Build history of the part. All positions in model axes, mm. A direction names the side the tool comes from. Give positions to 0.01 mm unless a question says otherwise; leave off trailing zeros. Write each loop counter-clockwise with the first axis right and the second up, starting at its lowest first coordinate (ties: lowest second). Pieces come first, ordered by that corner, then holes. Notation, with made-up numbers: M -13,81 L 37,81 A18 ccw 37,88 Z; hole C 88,76 d8. An arc over 180 degrees is marked long. Return JSON: item names as keys, results as strings. Group by question number.
Q1. Band-saw the part on B-B, the plane x = 0. Give the cut face in (y, z).
Q2. Band-saw the part on C-C, the plane z = -0.65. Give the cut face in (x, y).
Q3. Band-saw the part on A-A, the plane y = -22.5. Give the cut face in (x, z).
Q4. Tool access for faces 1 (the flat face through (0, 0, 0)), 2 (the cylindrical face through (0.45, -2.37, 1.43)): list every direction of +Z, -Z, +X, -X, +Y, -Y with a clear straight run to the whole face (end or side of a thin tool).
Q5. Flat gauge pins, fed straight in: pin 1 Ø0.7 at (x, y) = (-1, -19) entering from +Z; pin 2 Ø0.7 at (x, y) = (-1, -21.5) entering from -Z. Where does each tip first touch, or does it go through?
Q6. Wall check: probe 1 along Z at (x, y) = (1, -11.5); probe 2 along Y at (x, z) = (0.2, -0.85); probe 3 along Y at (x, z) = (-0.3, -1.5). Give the ranges that are in metal, low to high.
from build123d import *

# Parameters (mm, degrees)
SKETCH1_R           = 1.5
BOSS_EXTRUDE1_DEPTH = 4.8
SKETCH2_R           = 1.7
BOSS_EXTRUDE2_DEPTH = 1.2
SKETCH3_W           = 0.6
SKETCH3_H           = 0.4
BOSS_EXTRUDE3_DEPTH = 27


with BuildPart() as part:
    # Sketch1 → Boss-Extrude1 (new body)
    with BuildSketch(Plane(origin=(0, 0, 0), x_dir=(1, 0, 0), z_dir=(0, 1, 0))):
        with Locations(Location((0, 0, 0), (0, 0, 270))):
            Circle(SKETCH1_R)
    extrude(amount=-BOSS_EXTRUDE1_DEPTH)

    # Sketch2 → Boss-Extrude2 (add)
    with BuildSketch(Plane.XZ.offset(4.8)):
        with Locations(Location((0, 0, 0), (0, 0, 270))):
            Circle(SKETCH2_R)
    extrude(amount=BOSS_EXTRUDE2_DEPTH)

    # Sketch3 → Boss-Extrude3 (add)
    with BuildSketch(Plane.XZ.offset(6)):
        with Locations((-1.27, 0)):
            Rectangle(SKETCH3_W, SKETCH3_H)
        with Locations((1.27, 0)):
            Rectangle(SKETCH3_W, SKETCH3_H)
    extrude(amount=BOSS_EXTRUDE3_DEPTH)


solid = part.part
From the geometry:
{
 "1": {"outline": "M -6,-1.7 L -4.8,-1.7 L -4.8,-1.5 L 0,-1.5 L 0,1.5 L -4.8,1.5 L -4.8,1.7 L -6,1.7 Z"},
 "2": {"outline": "M -1.57,-6 L 1.57,-6 L 1.57,-4.8 L 1.35,-4.8 L 1.35,0 L -1.35,0 L -1.35,-4.8 L -1.57,-4.8 Z"},
 "3": {"outline": "M -1.57,-0.2 L -0.97,-0.2 L -0.97,0.2 L -1.57,0.2 Z; M 0.97,-0.2 L 1.57,-0.2 L 1.57,0.2 L 0.97,0.2 Z"},
 "4": {"face 1": "+Z, -Z, +X, -X, +Y", "face 2": "+Y"},
 "5": {"pin 1": "stops at z = 0.2", "pin 2": "stops at z = -0.2"},
 "6": {"probe 1": "z = -0.2 to 0.2", "probe 2": "y = -6 to 0", "probe 3": "y = -6 to -4.8"}
}
